from build123d import *

# Parameters (mm, degrees)
F0_W     = 35.56
F0_H     = 16.002
F1_DEPTH = 1.27
F3_D     = 7.8994
F4_DEPTH = 1.271


with BuildPart() as f1:
    # F0 (on Top) → F1 (new body)
    with BuildSketch(Plane.XY):
        Rectangle(F0_W, F0_H)
    extrude(amount=F1_DEPTH)

    # F3 (through all)
    with Locations(Plane(origin=(0, 0, 0), x_dir=(1, 0, 0), z_dir=(0, 0, -1))):
        with Locations((2.286, 0)):
            Hole(F3_D / 2)

    # F2 (on face) → F4 (cut, through all)
    with BuildSketch(Plane(origin=(0, 0, 0), x_dir=(1, 0, 0), z_dir=(0, 0, -1))):
        Polygon((-12.55014, 3.81), (-12.55014, 0), (-8.74014, 0), (-4.93014, 0), (-4.93014, 3.81), align=None)
        Polygon((-8.74014, 0), (-12.55014, 0), (-12.55014, -3.81), (-4.93014, -3.81), (-4.93014, 0), align=None)
    extrude(amount=-F4_DEPTH, mode=Mode.SUBTRACT)


solid = f1.part
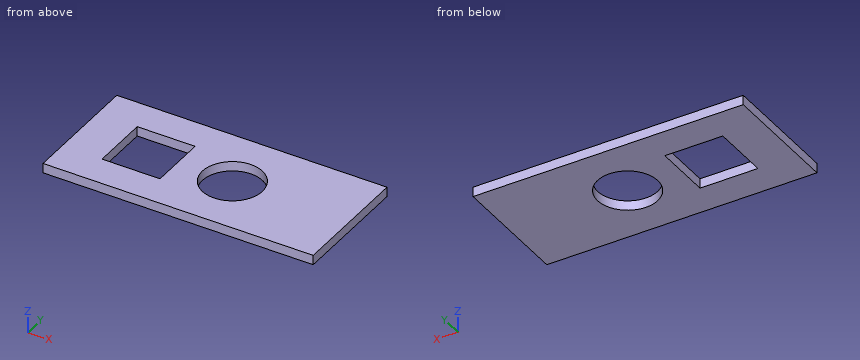
Design review of the part built by this model. Coordinates are the model's own, in mm. Give positions to 0.01 mm unless a question says otherwise; leave off trailing zeros. Order: outer loops, then holes, each group sorted by start corner. A loop starts at its lowest first (then second) coordinate and runs counter-clockwise, first axis right, second up. Notation, with made-up numbers: (59, -20.5) - (73, -20.5) arc R20 cw to (73, -15.5) - close; hole circle Ø6 at (-26.75, 21.25). An arc over 180 degrees is marked (long way). Write item = value, one per line. Start each with the question number.
Q1. We need section B-B on x = -12. State the section outline as (y, z) points.
Q2. We need section A-A on y = 0. State the section outline as (x, z) points, plus the area to 3 significant figures.
Q3. To check wall thickness, follow L1, parallel to Y at x = -7, z = 0.65; L2, parallel to X at y = 1.5, z = 0.9; L3, parallel to X at y = -2.5, z = 0.75. State the ranges of each line that lie inside material, in increasing order. Write a range as from..to.
Q4. We need section C-C on z = 0.85. State the section outline as (x, y) points.
Q5. We need section D-D on x = 5.5. State the section outline as (y, z) points, plus the area to 3 significant figures.
Working result:
q1.outline = (-8, 0) - (-3.81, 0) - (-3.81, 1.27) - (-8, 1.27) - close; (3.81, 0) - (8, 0) - (8, 1.27) - (3.81, 1.27) - close
q2.outline = (-17.78, 0) - (-12.55, 0) - (-12.55, 1.27) - (-17.78, 1.27) - close; (-4.93, 0) - (-1.66, 0) - (-1.66, 1.27) - (-4.93, 1.27) - close; (6.24, 0) - (17.78, 0) - (17.78, 1.27) - (6.24, 1.27) - close
q2.area = 25.5 mm²
q3.L1 = -8..-3.81, 3.81..8
q3.L2 = -17.78..-12.55, -4.93..-1.37, 5.94..17.78
q3.L3 = -17.78..-12.55, -4.93..-0.77, 5.34..17.78
q4.outline = (-17.78, -8) - (17.78, -8) - (17.78, 8) - (-17.78, 8) - close; hole (-12.55, -3.81) - (-4.93, -3.81) - (-4.93, 3.81) - (-12.55, 3.81) - close; hole circle Ø7.9 at (2.29, 0)
q5.outline = (-8, 0) - (-2.3, 0) - (-2.3, 1.27) - (-8, 1.27) - close; (2.3, 0) - (8, 0) - (8, 1.27) - (2.3, 1.27) - close
q5.area = 14.5 mm²
